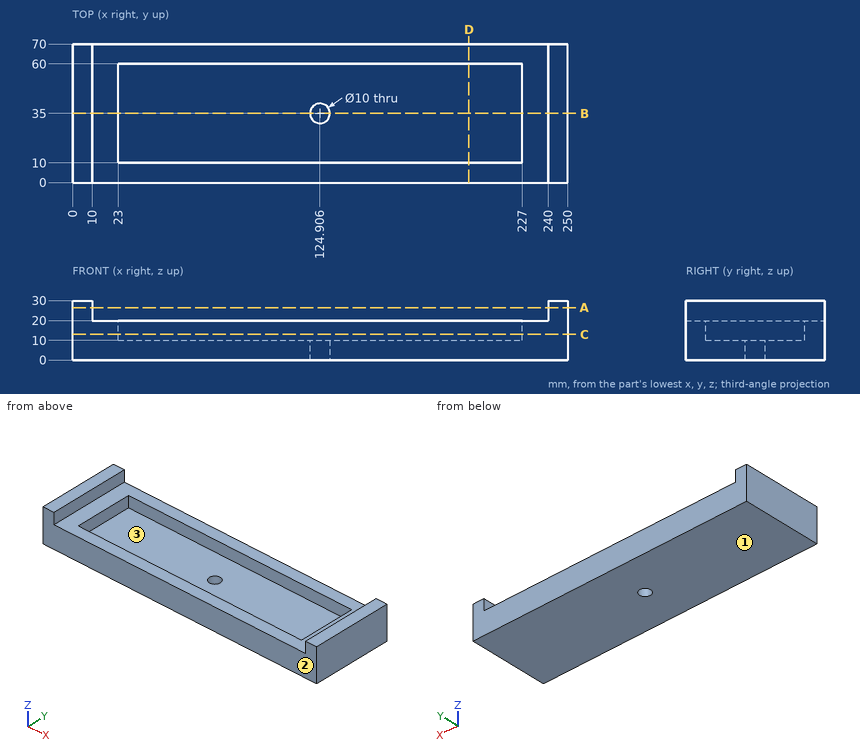
Input: dimensioned drawing with shaded views. Units: mm. Origin: part minimum x, y, z. Coordinates: 2 decimals unless noted, no trailing zeros. Write each loop counter-clockwise with the first axis right and the second up, starting at its lowest first coordinate (ties: lowest second). Pieces come first, ordered by that corner, then holes. Notation, with made-up numbers: M -22,6.25 L 14,6.25 A25 cw 14,39.25 Z; hole C 78.5,-7.75 d8. An arc over 180 degrees is marked long. Answer as a JSON object with one key per item and string values. Group by question number.
(1) Contact query for flat-ended pins moving along their axis: P1, Ø12, axis at y = 8, z = 8.5, coming from the -X side; P2, Ø15, axis at x = 102.5, y = 39, coming from the +Z side. Output: stop coordinate, or through.
(2) Section C-C on z = 13. Output: boundary loops of the cut face in (x, y).
(3) Section A-A on z = 26.5. Output: boundary loops of the cut face in (x, y).
(4) Ray query, line 1 along X through (y, z) = (32, 14.5); line 2 along Y through (x, z) = (176, 16); line 3 along X through (y, z) = (33.5, 22). Return the intervals inside material, ascending. Write a range as [from, to].
(5) Section B-B on y = 35. Output: boundary loops of the cut face in (x, z).
(6) Section D-D on x = 200. Output: boundary loops of the cut face in (y, z).
(7) Mould query, pull axis Z, two halves, no side actions, for the marked faces 1, 2 and 3. Classes: pulls with the +Z half, pulls with the -Z half, needs draft (parallel to the pull), parting line crosses it, or undercut.
Result set:
{
 "1": {"P1": "stops at x = 0", "P2": "stops at z = 10"},
 "2": {"outline": "M 0,0 L 250,0 L 250,70 L 0,70 Z; hole M 23,10 L 227,10 L 227,60 L 23,60 Z"},
 "3": {"outline": "M 0,0 L 10,0 L 10,70 L 0,70 Z; M 240,0 L 250,0 L 250,70 L 240,70 Z"},
 "4": {"line 1": "x = [0, 23], [227, 250]", "line 2": "y = [0, 10], [60, 70]", "line 3": "x = [0, 10], [240, 250]"},
 "5": {"outline": "M 0,0 L 119.91,0 L 119.91,10 L 23,10 L 23,20 L 10,20 L 10,30 L 0,30 Z; M 129.91,0 L 250,0 L 250,30 L 240,30 L 240,20 L 227,20 L 227,10 L 129.91,10 Z"},
 "6": {"outline": "M 0,0 L 70,0 L 70,20 L 60,20 L 60,10 L 10,10 L 10,20 L 0,20 Z"},
 "7": {"face 1": "pulls with the -Z half", "face 2": "needs draft", "face 3": "pulls with the +Z half"}
}
